Model file for the job. Use its own axes, mm. Give positions to 0.01 mm unless a question says otherwise; leave off trailing zeros. Loops run counter-clockwise (first coordinate to the right, second up) from the corner with the lowest first, then second, coordinate; pieces in that order, holes last. Notation, with made-up numbers: (72.25, -23) - (120.25, -23) arc R19 ccw to (120.25, -5) - close; hole circle Ø6 at (31, 32). An arc over 180 degrees is marked (long way). Use a Markdown table: item, result.
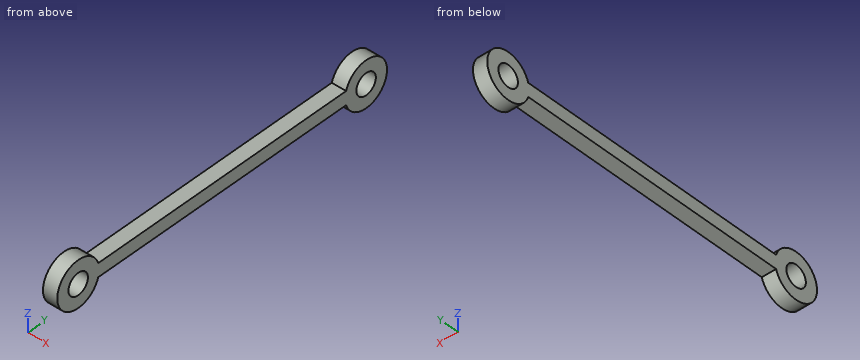
from build123d import *

# Parameters (mm, degrees)
F0_R     = 7.201014
F1_DEPTH = 4.826


with BuildPart() as f1:
    # F0 (on Right) → F1 (new body)
    with BuildSketch(Plane.YZ):
        with BuildLine():
            Line((0, -4.541845), (0, 4.541845))
            Line((0, 4.541845), (-91.654071, 4.541845))
            ThreePointArc((-91.654071, 4.541845), (-121.932156, 0), (-91.654071, -4.541845))
            Line((-91.654071, -4.541845), (0, -4.541845))
        make_face()
        with Locations((-106.452465, 0)):
            Circle(F0_R, mode=Mode.SUBTRACT)
    extrude(amount=F1_DEPTH)

    # F2: F1 across plane


with BuildPart() as f1_1:
    add(f1.part)
    add(f1.part.mirror(Plane.YZ))

    # F3: F1 across plane


with BuildPart() as f1_2:
    add(f1_1.part)
    add(f1_1.part.mirror(Plane.XZ))


solid = f1_2.part
(1) Slice it at B-B, the plane x = -1.25. Write the cut outline in (y, z), plus the area to 3 significant figures.
Computed:
| item | result |
|---|---|
| outline | (-91.65, -4.54) - (91.65, -4.54) arc R15.48 ccw (long way) to (91.65, 4.54) - (-91.65, 4.54) arc R15.48 ccw (long way) to start; hole circle Ø14.4 at (-106.45, 0); hole circle Ø14.4 at (106.45, 0) |
| area | 2,840 mm² |
(2) Slice it at D-D, the plane y = -102.5. Write the cut outline in (x, z).
Computed:
| item | result |
|---|---|
| outline | (-4.83, -14.97) - (4.83, -14.97) - (4.83, -6.02) - (-4.83, -6.02) - close; (-4.83, 6.02) - (4.83, 6.02) - (4.83, 14.97) - (-4.83, 14.97) - close |
(3) Slice it at A-A, the plane z = 0. Write the cut outline in (x, y), plus the area to 3 significant figures.
Computed:
| item | result |
|---|---|
| outline | (-4.83, -121.93) - (4.83, -121.93) - (4.83, -113.65) - (-4.83, -113.65) - close; (-4.83, -99.25) - (4.83, -99.25) - (4.83, 99.25) - (-4.83, 99.25) - close; (-4.83, 113.65) - (4.83, 113.65) - (4.83, 121.93) - (-4.83, 121.93) - close |
| area | 2,080 mm² |
(4) Drill centre lines: probe 1 along Y at (x, z) = (-0.5, 6); probe 2 along Y at (x, z) = (-2.25, 1); probe 3 along Y at (x, z) = (1.75, 13.5). Where is each one in solid material? Low to high. Write a range as [from, to].
Computed:
| item | result |
|---|---|
| probe 1 | [-120.72, -110.43], [-102.47, -92.18], [92.18, 102.47], [110.43, 120.72] |
| probe 2 | [-121.9, -113.58], [-99.32, 99.32], [113.58, 121.9] |
| probe 3 | [-114.03, -98.88], [98.88, 114.03] |
(5) Pin check, flat tips, straight feed: P1, Ø5, axis at x = -2, z = 12, coming from the -Y side; P2, Ø1.5, axis at x = 3.5, y = 22, coming from the +Z side; P3, Ø5, axis at x = 1, z = 3.5, coming from the +Y side. Stop position of each tip, or through.
Computed:
| item | result |
|---|---|
| P1 | y = -118.67 |
| P2 | z = 4.54 |
| P3 | y = 121.9 |
(6) Slice it at C-C, the plane z = 11. Write the cut outline in (x, y).
Computed:
| item | result |
|---|---|
| outline | (-4.83, -117.34) - (4.83, -117.34) - (4.83, -95.56) - (-4.83, -95.56) - close; (-4.83, 95.56) - (4.83, 95.56) - (4.83, 117.34) - (-4.83, 117.34) - close |
